Here's the drawing with two shaded views (mm, measured from the low corner). I have some questions. A direction names the side the tool comes from. Give positions to 0.01 mm unless a question says otherwise; leave off trailing zeros. Write each loop counter-clockwise with the first axis right and the second up, starting at its lowest first coordinate (ties: lowest second). Pieces come first, ordered by that corner, then holes. Notation, with made-up numbers: M 41.5,23.25 L 69.5,23.25 A19 ccw 69.5,38.25 Z; hole C 42,49.5 d11. An arc over 180 degrees is marked long. Use one line per item in the form item = value. Start each with the question number.
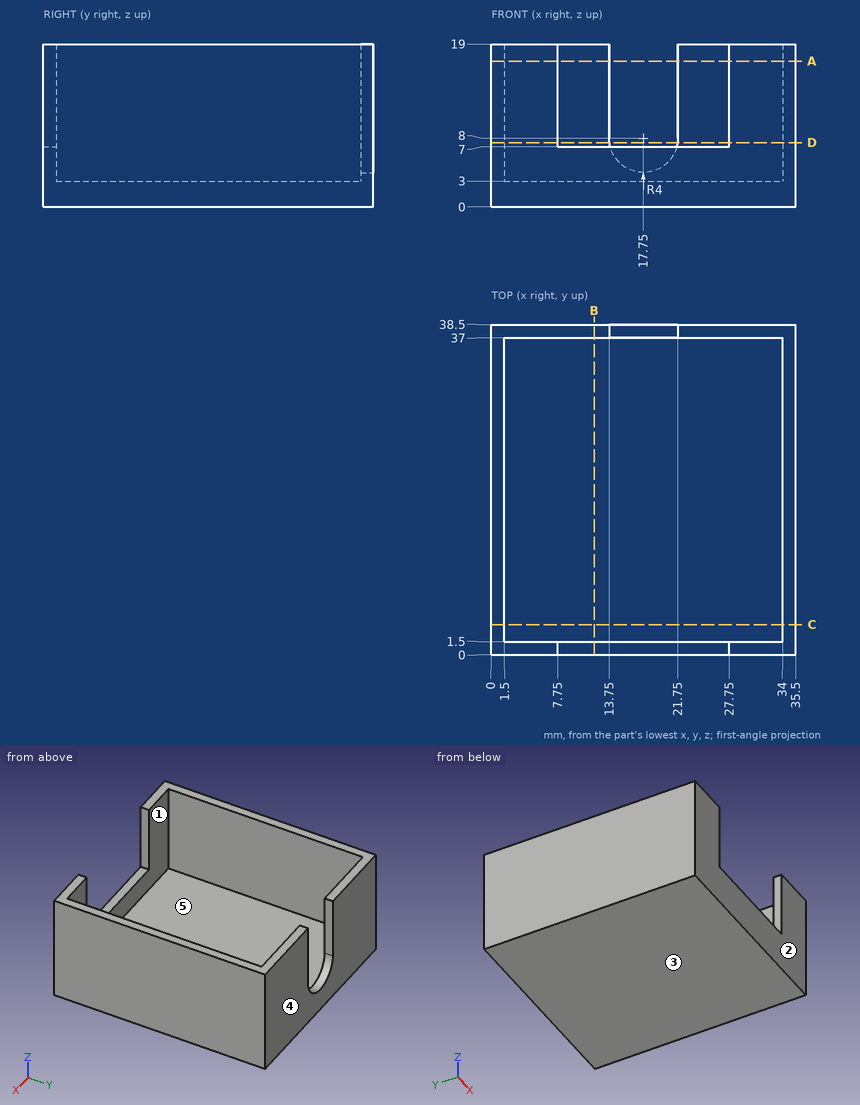
1) Please list where these lines run through material, in increasing order: line 1 (X direction, y = 16, z = 12.25); line 2 (Y direction, x = 3, z = 4); line 3 (Z direction, x = 20, y = 36.5).
2) Suppose I cut it at A-A, the plane z = 17. List the corners of the cut face in (x, y) for me.
3) Suppose I cut it at B-B, the plane x = 12. List the corners of the cut face in (y, z) for me, and give its area (4 significant figures).
4) Suppose I cut it at D-D, the plane z = 7.5. List the corners of the cut face in (x, y) for me.
5) Will these pins go through, and if not, where does the flat tip stop? P1, Ø5, axis at x = 23.5, y = 28, coming from the +Z side; P2, Ø1.6, axis at x = 16.5, y = 0.5, coming from the +Z side.
6) Thinking about a two-plate mould opening in Y: for the marked faces 1, 2 and 3, which applies, released by +Y, released by -Y, zero draft, split by the parting line, or undercut?
7) Suppose I cut it at C-C, the plane y = 3.5. List the corners of the cut face in (x, z) for me.
8) On a 3-axis mill with a long thin cutter (end or side, diameter ignored), from which of +Z, -Z, +X, -X, +Y, -Y can I reach the whole of each face in a straight line? I mean the marked faces 4 and 5. Say none if no direction works.
Checks:
q1.line_1 = 0 to 1.5, 34 to 35.5
q1.line_2 = 0 to 1.5, 37 to 38.5
q1.line_3 = 0 to 3
q2.outline = M 0,0 L 7.75,0 L 7.75,1.5 L 1.5,1.5 L 1.5,37 L 13.75,37 L 13.75,38.5 L 0,38.5 Z; M 21.75,37 L 34,37 L 34,1.5 L 27.75,1.5 L 27.75,0 L 35.5,0 L 35.5,38.5 L 21.75,38.5 Z
q3.outline = M 0,0 L 38.5,0 L 38.5,19 L 37,19 L 37,3 L 1.5,3 L 1.5,7 L 0,7 Z
q3.area = 145.5 mm^2
q4.outline = M 0,0 L 7.75,0 L 7.75,1.5 L 1.5,1.5 L 1.5,37 L 13.78,37 L 13.78,38.5 L 0,38.5 Z; M 21.72,37 L 34,37 L 34,1.5 L 27.75,1.5 L 27.75,0 L 35.5,0 L 35.5,38.5 L 21.72,38.5 Z
q5.P1 = 3
q5.P2 = 7
q6.face_1 = undercut
q6.face_2 = released by -Y
q6.face_3 = zero draft
q7.outline = M 0,0 L 35.5,0 L 35.5,19 L 34,19 L 34,3 L 1.5,3 L 1.5,19 L 0,19 Z
q8.face_4 = +Z, -Z, +X, -X, +Y
q8.face_5 = +Z
